from build123d import *

# Parameters (mm, degrees)
F0_W     = 225.425
F0_H     = 57.15
F1_DEPTH = 6.35
F3_DEPTH = 12.701


with BuildPart() as f1:
    # F0 (on Front) → F1 (new body, symmetric)
    with BuildSketch(Plane.XZ):
        Rectangle(F0_W, F0_H)
    extrude(amount=F1_DEPTH, both=True)

    # F2 (on face) → F3 (cut, through all)
    with BuildSketch(Plane.XZ.offset(6.35)):
        with BuildLine():
            Line((-84.1344035983, 6.3598155975), (-106.3594035983, 6.3598155975))
            ThreePointArc((-106.3594035983, 6.3598155975), (-95.2469035983, -4.7526844025), (-84.1344035983, 6.3598155975))
        make_face()
        with BuildLine():
            ThreePointArc((-84.1344035983, 6.3598155975), (-95.2469035983, 17.4723155975), (-106.3594035983, 6.3598155975))
            Line((-106.3594035983, 6.3598155975), (-84.1344035983, 6.3598155975))
        make_face()
        with BuildLine():
            Line((-20.6365519956, 6.359861698), (-42.8615519956, 6.359861698))
            ThreePointArc((-42.8615519956, 6.359861698), (-31.7490519956, -4.752638302), (-20.6365519956, 6.359861698))
        make_face()
        with BuildLine():
            ThreePointArc((-20.6365519956, 6.359861698), (-31.7490519956, 17.472361698), (-42.8615519956, 6.359861698))
            Line((-42.8615519956, 6.359861698), (-20.6365519956, 6.359861698))
        make_face()
        with BuildLine():
            Line((42.8613498986, 6.3600256108), (20.6363498986, 6.3600256108))
            ThreePointArc((20.6363498986, 6.3600256108), (31.7488498986, -4.7524743892), (42.8613498986, 6.3600256108))
        make_face()
        with BuildLine():
            ThreePointArc((42.8613498986, 6.3600256108), (31.7488498986, 17.4725256108), (20.6363498986, 6.3600256108))
            Line((20.6363498986, 6.3600256108), (42.8613498986, 6.3600256108))
        make_face()
        with BuildLine():
            Line((106.3594967306, 6.360122934), (84.1344967306, 6.360122934))
            ThreePointArc((84.1344967306, 6.360122934), (95.2469967306, -4.752377066), (106.3594967306, 6.360122934))
        make_face()
        with BuildLine():
            ThreePointArc((106.3594967306, 6.360122934), (95.2469967306, 17.472622934), (84.1344967306, 6.360122934))
            Line((84.1344967306, 6.360122934), (106.3594967306, 6.360122934))
        make_face()
    extrude(amount=-F3_DEPTH, mode=Mode.SUBTRACT)


solid = f1.part
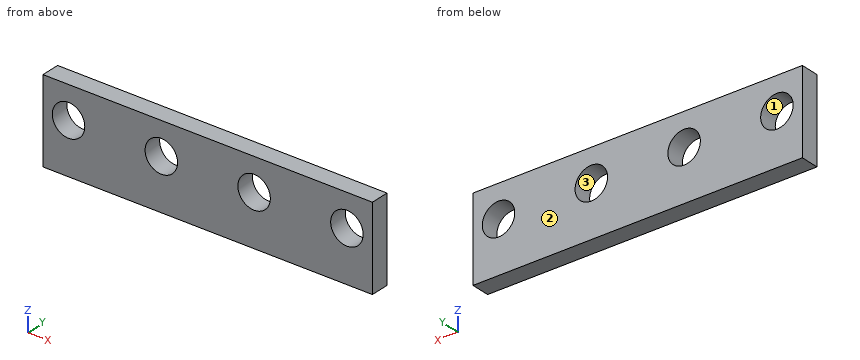
Check sheet for the modelled part. Datum: model origin and axes. Units: mm. Face numbers are marked on the shaded views. Round coordinates to 2 decimals unless told otherwise and drop trailing zeros. Write each loop counter-clockwise with the first axis right and the second up, starting at its lowest first coordinate (ties: lowest second). Pieces come first, ordered by that corner, then holes. Notation, with made-up numbers: (26.25, -26) -> (79.25, -26) arc R13 cw to (79.25, -3) -> close; hole circle Ø2 at (37.25, -9.5). An arc over 180 degrees is marked (long way). Answer as CSV lines item,"result". Start each with the question number.
1) Go/stop test with a flat-tipped pin: P1, Ø20, axis at x = 95.25, z = 6.36, coming from the +Y side. Record where the tip stops, or that it passes through.
2) Section check C-C on y = 4.25. Enter the section's corners in (x, z) (1 decimal), and give its area (3 significant figures).
3) Section check B-B on x = -39. Enter the section's corners in (y, z) (3 decimals).
4) Material ranges on line 1 (X direction, y = -3.5, z = 15); line 2 (X direction, y = 4, z = 11); line 3 (Z direction, x = -89, y = -2) (3 decimals), recorded low to high. Write a range as from..to.
5) Release check for a two-part mould opening along Z. For the marked faces 1, 2 and 3 record: pulls with the +Z half, pulls with the -Z half, needs draft (parallel to the pull), parting line crosses it, or undercut.
6) Section check A-A on z = 0. Enter the section's corners in (x, y), and give its area (3 significant figures).
7) Section check D-D on x = 36. Enter the section's corners in (y, z) (3 decimals), and give its area (3 significant figures).
Found:
1,P1,"passes through"
2,outline,"(-112.7, -28.6) -> (112.7, -28.6) -> (112.7, 28.6) -> (-112.7, 28.6) -> close; hole circle Ø22.2 at (-95.2, 6.4); hole circle Ø22.2 at (-31.7, 6.4); hole circle Ø22.2 at (31.7, 6.4); hole circle Ø22.2 at (95.2, 6.4)"
2,area,"11,300 mm^2"
3,outline,"(-6.35, -28.575) -> (6.35, -28.575) -> (6.35, -2.061) -> (-6.35, -2.061) -> close; (-6.35, 14.781) -> (6.35, 14.781) -> (6.35, 28.575) -> (-6.35, 28.575) -> close"
4,line 1,"x = -112.71..-102.24, -88.26..-38.74, -24.76..24.76, 38.74..88.26, 102.24..112.71"
4,line 2,"x = -112.71..-105.34, -85.15..-41.85, -21.65..21.65, 41.85..85.15, 105.34..112.71"
4,line 3,"z = -28.575..-2.831, 15.55..28.575"
5,face 1,"undercut"
5,face 2,"needs draft"
5,face 3,"undercut"
6,outline,"(-112.71, -6.35) -> (-104.36, -6.35) -> (-104.36, 6.35) -> (-112.71, 6.35) -> close; (-86.13, -6.35) -> (-40.86, -6.35) -> (-40.86, 6.35) -> (-86.13, 6.35) -> close; (-22.64, -6.35) -> (22.64, -6.35) -> (22.64, 6.35) -> (-22.64, 6.35) -> close; (40.86, -6.35) -> (86.13, -6.35) -> (86.13, 6.35) -> (40.86, 6.35) -> close; (104.36, -6.35) -> (112.71, -6.35) -> (112.71, 6.35) -> (104.36, 6.35) -> close"
6,area,"1,940 mm^2"
7,outline,"(-6.35, -28.575) -> (6.35, -28.575) -> (6.35, -3.907) -> (-6.35, -3.907) -> close; (-6.35, 16.627) -> (6.35, 16.627) -> (6.35, 28.575) -> (-6.35, 28.575) -> close"
7,area,"465 mm^2"
